Can you work these out from the model? Positions are in its coordinate system, mm. Give positions to 0.01 mm unless a question says otherwise; leave off trailing zeros. Write each loop counter-clockwise with the first axis right and the second up, starting at its lowest first coordinate (ties: lowest second). Pieces come first, ordered by that corner, then holes. Notation, with made-up numbers: M -32.5,8 L -13.5,8 A28 ccw -13.5,47 Z; hole C 50,-18.5 d5. An arc over 180 degrees is marked long. Use CSV: the item, a comma, the result in double quotes. Start each with the question number.
from build123d import *

# Parameters (mm, degrees)
SKETCH_1_W      = 70.11
SKETCH_1_H      = 85.3
EXTRUDE_1_DEPTH = 0.5
SKETCH_1_3_W    = 68.11
SKETCH_1_3_H    = 81.3
EXTRUDE_2_DEPTH = 0.7
FILLET_1_R      = 1.4
FILLET_2_R      = 1.4
SKETCH_1_4_W    = 13
SKETCH_1_4_H    = 4.5
EXTRUDE_3_DEPTH = 1


with BuildPart() as part:
    # 草图1 → 凸台-拉伸1 (new body)
    with BuildSketch(Plane.XY):
        with Locations((-3.095661812, -6.162041577)):
            Rectangle(SKETCH_1_W, SKETCH_1_H)
    extrude(amount=EXTRUDE_1_DEPTH)

    # 草图1<3> → 凸台-拉伸2 (add)
    with BuildSketch(Plane.XY):
        with Locations((-3.095661812, -6.162041577)):
            Rectangle(SKETCH_1_3_W, SKETCH_1_3_H)
    extrude(amount=-EXTRUDE_2_DEPTH)

    # 圆角1
    fillet_1_edges = [part.edges().sort_by_distance(p)[0] for p in [
        (-37.150661812, -46.812041577, -0.35),
        (-37.150661812, 34.487958423, -0.35),
        (30.959338188, 34.487958423, -0.35),
        (30.959338188, -46.812041577, -0.35),
    ]]
    fillet(fillet_1_edges, radius=FILLET_1_R)

    # 圆角2
    fillet_2_edges = [part.edges().sort_by_distance(p)[0] for p in [
        (-38.150661812, 36.487958423, 0.25),
        (31.959338188, 36.487958423, 0.25),
        (31.959338188, -48.812041577, 0.25),
        (-38.150661812, -48.812041577, 0.25),
    ]]
    fillet(fillet_2_edges, radius=FILLET_2_R)

    # 草图1<4> → 凸台-拉伸3 (add)
    with BuildSketch(Plane.XY):
        with Locations((-12.141661812, 12.437958423)):
            Rectangle(SKETCH_1_4_W, SKETCH_1_4_H)
    extrude(amount=-EXTRUDE_3_DEPTH)


solid = part.part
(1) I want a section at A-A (x = -28). Write out the boundary of the cut face in (y, z), and give its area (3 significant figures).
(2) Will this pin go through, and if not, where does the flat tip stop? pin 1 Ø20.5 at (x, y) = (-2.5, -24) entering from -Z.
(3) I want a section at C-C (x = -7). Write out the boundary of the cut face in (y, z), and give its area (3 significant figures).
(4) Please list where these lines run through material, in increasing order: L1, parallel to X at y = 1.5, z = -0.45; L2, parallel to Y at x = 5, z = -0.5; L3, parallel to Z at x = 23.5, y = -30.5. Write a range as [from, to].
(5) I want a section at B-B (y = -30). Write out the boundary of the cut face in (x, z), and give its area (3 significant figures).
Geometry results:
1,outline,"M -48.81,0 L -46.81,0 L -46.81,-0.7 L 34.49,-0.7 L 34.49,0 L 36.49,0 L 36.49,0.5 L -48.81,0.5 Z"
1,area,"99.6 mm2"
2,pin 1,"stops at z = -0.7"
3,outline,"M -48.81,0 L -46.81,0 L -46.81,-0.7 L 10.19,-0.7 L 10.19,-1 L 14.69,-1 L 14.69,-0.7 L 34.49,-0.7 L 34.49,0 L 36.49,0 L 36.49,0.5 L -48.81,0.5 Z"
3,area,"101 mm2"
4,L1,"x = [-37.15, 30.96]"
4,L2,"y = [-46.81, 34.49]"
4,L3,"z = [-0.7, 0.5]"
5,outline,"M -38.15,0 L -37.15,0 L -37.15,-0.7 L 30.96,-0.7 L 30.96,0 L 31.96,0 L 31.96,0.5 L -38.15,0.5 Z"
5,area,"82.7 mm2"
